Read the model definition and answer for the solid it produces. Units are mm, in the model's axes. Face numbers are marked on the shaded views. A direction names the side the tool comes from. Round coordinates to 2 decimals unless told otherwise and drop trailing zeros. Loops run counter-clockwise (first coordinate to the right, second up) from the corner with the lowest first, then second, coordinate; pieces in that order, holes last. Notation, with made-up numbers: M -36,79 L 16,79 A22 ccw 16,86 Z; hole C -7.75,19.5 d3. An arc over 180 degrees is marked long. Answer as CSV lines item,"result".
```python
from build123d import *

# Parameters (mm, degrees)
SKETCH1_W      = 410
SKETCH1_H      = 120
SKETCH1_R      = 15.5
EXTRUDE1_DEPTH = 12
SKETCH2_W      = 410
SKETCH2_H      = 12
EXTRUDE2_DEPTH = 398
SKETCH3_R      = 15.5
EXTRUDE3_DEPTH = 198
SKETCH4_W      = 12
SKETCH4_H      = 96
EXTRUDE4_DEPTH = 188
EXTRUDE5_DEPTH = 188


with BuildPart() as part:
    # Sketch1 → Extrude1 (new body)
    with BuildSketch(Plane.XY):
        with Locations((205, 60)):
            Rectangle(SKETCH1_W, SKETCH1_H)
        with Locations((45, 67)):
            Circle(SKETCH1_R, mode=Mode.SUBTRACT)
        with Locations((145, 67)):
            Circle(SKETCH1_R, mode=Mode.SUBTRACT)
        with Locations((365, 67)):
            Circle(SKETCH1_R, mode=Mode.SUBTRACT)
        with Locations((265, 67)):
            Circle(SKETCH1_R, mode=Mode.SUBTRACT)
    extrude(amount=EXTRUDE1_DEPTH)

    # Sketch2 → Extrude2 (add)
    with BuildSketch(Plane.XY.offset(12)):
        with Locations((205, 6)):
            Rectangle(SKETCH2_W, SKETCH2_H)
    extrude(amount=EXTRUDE2_DEPTH)

    # Sketch3 → Extrude3 (cut)
    with BuildSketch(Plane(origin=(0, 12, 0), x_dir=(1, 0, 0), z_dir=(0, 1, 0))):
        with BuildLine():
            add(Edge.make_bspline(
                [(205, -410), (307.5, -410), (410, -210)],
                knots=[0.5, 0.5, 0.5, 1, 1, 1], degree=2))
            Line((205, -410), (410, -410))
            Line((410, -410), (410, -210))
        make_face()
        with BuildLine():
            add(Edge.make_bspline(
                [(0, -210), (102.5, -410), (205, -410)],
                knots=[0, 0, 0, 0.5, 0.5, 0.5], degree=2))
            Line((0, -210), (0, -410))
            Line((0, -410), (205, -410))
        make_face()
        with Locations(Location((107.261778202, -121.586347917, 0), (0, 0, 270))):
            Circle(SKETCH3_R)
        with Locations(Location((205, -364, 0), (0, 0, 270))):
            Circle(SKETCH3_R)
        with Locations(Location((50.874342549, -191.732317869, 0), (0, 0, 270))):
            Circle(SKETCH3_R)
        with Locations(Location((205, -274, 0), (0, 0, 270))):
            Circle(SKETCH3_R)
        with Locations(Location((359.125657451, -191.732317869, 0), (0, 0, 270))):
            Circle(SKETCH3_R)
        with Locations(Location((302.738221798, -121.586347917, 0), (0, 0, 270))):
            Circle(SKETCH3_R)
    extrude(amount=-EXTRUDE3_DEPTH, mode=Mode.SUBTRACT)

    # Sketch4 → Extrude4 (add)
    with BuildSketch(Plane.XY.offset(12)):
        with Locations((205, 60)):
            Rectangle(SKETCH4_W, SKETCH4_H)
    extrude(amount=EXTRUDE4_DEPTH)

    # Sketch5 → Extrude5 (cut)
    with BuildSketch(Plane.ZY.offset(-199)):
        Polygon((200, 108), (200, 24), (24, 108), align=None)
    extrude(amount=-EXTRUDE5_DEPTH, mode=Mode.SUBTRACT)


solid = part.part
```
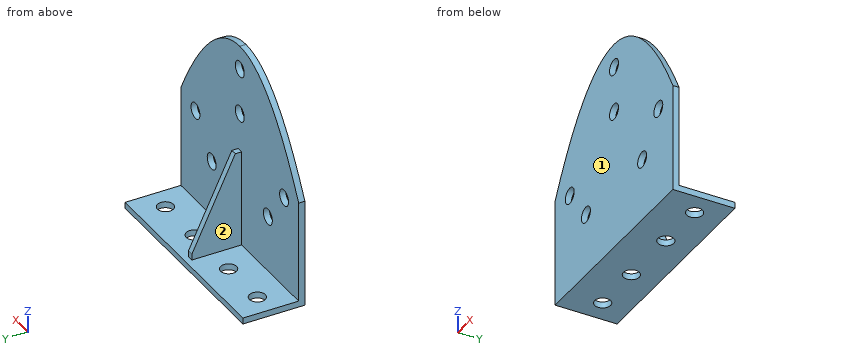
1) Find section C-C, the plane y = 35. Give the vertices of the cut face in (x, z).
Evaluation:
outline,"M 0,0 L 410,0 L 410,12 L 211,12 L 211,176.95 L 199,176.95 L 199,12 L 0,12 Z"
2) Each of these flat-tipped pins is pushed along its axis until it touches: P1, Ø10, axis at x = 153.5, z = 104, coming from the -Y side; P2, Ø1.5, axis at x = 222, z = 328, coming from the +Y side; P3, Ø9.5, axis at x = 203, y = 17, coming from the +Z side; P4, Ø1.5, axis at x = 161.5, y = 104, coming from the +Z side. Where does it stop, or does it pass through?
Evaluation:
P1,"stops at y = 0"
P2,"stops at y = 12"
P3,"stops at z = 200"
P4,"stops at z = 12"
3) Find section B-B, the plane z = 183. Give the vertices of the cut face in (x, y).
Evaluation:
outline,"M 0,0 L 38.07,0 L 38.07,12 L 0,12 Z; M 63.68,0 L 346.32,0 L 346.32,12 L 211,12 L 211,32.11 L 199,32.11 L 199,12 L 63.68,12 Z; M 371.93,0 L 410,0 L 410,12 L 371.93,12 Z"
4) Find section D-D, the plane z = 63. Give the vertices of the cut face in (x, y), then the cut area to 3 significant figures.
Evaluation:
outline,"M 0,0 L 410,0 L 410,12 L 211,12 L 211,89.39 L 199,89.39 L 199,12 L 0,12 Z"
area,"5,850 mm^2"
5) Find section A-A, the plane y = 67. Give the vertices of the cut face in (x, z), then the cut area to 3 significant figures.
Evaluation:
outline,"M 0,0 L 29.5,0 L 29.5,12 L 0,12 Z; M 60.5,0 L 129.5,0 L 129.5,12 L 60.5,12 Z; M 160.5,0 L 249.5,0 L 249.5,12 L 211,12 L 211,109.9 L 199,109.9 L 199,12 L 160.5,12 Z; M 280.5,0 L 349.5,0 L 349.5,12 L 280.5,12 Z; M 380.5,0 L 410,0 L 410,12 L 380.5,12 Z"
area,"4,610 mm^2"
6) A tool of negligible diameter and unlimited length cuts with its end or side. For the marked faces 1 and 2, from which of +Z, -Z, +X, -X, +Y, -Y can it reach the whole face along a straight path? Write none if from no direction.
Evaluation:
face 1,"+Z, -Z, +X, -X, -Y"
face 2,"+Z, -X, +Y"
7) Straight lines are drawn through the part: line 1 (Y direction, x = 145, z = 5); line 2 (Z direction, x = 212, y = 22). For each, find the intervals that lie inside material, in ascending order.
Evaluation:
line 1,"y = 0 to 51.5, 82.5 to 120"
line 2,"z = 0 to 12"
